Design review of the part built by this model. Coordinates are the model's own, in mm. Round coordinates to 2 decimals unless told otherwise and drop trailing zeros. Loops run counter-clockwise (first coordinate to the right, second up) from the corner with the lowest first, then second, coordinate; pieces in that order, holes last. Notation, with made-up numbers: (-33.5, -16.75) - (-1.5, -16.75) arc R19 cw to (-1.5, 13.25) - close; hole circle Ø7 at (76.25, -3). An arc over 180 degrees is marked (long way). Return JSON: item names as keys, results as strings. Group by question number.
(1) We need section C-C, the plane x = 113. Write out the cut boundary in (y, z).
(2) Wall thickness on L1, parallel to X at y = 10, z = 149.5; L2, parallel to Z at x = 57.5, y = -54.5; L3, parallel to Z at x = 42, y = 3.5: over which ranges is each line inside the solid? List them lowest first. Write a range as [from, to].
(3) We need section A-A, the plane x = 33.5. Write out the cut boundary in (y, z).
(4) Clearance check with flat-ended pins moving along their axes: pin 1 (10 mm diameter, centred on x = 6, y = -2.5, fed in from +Z); pin 2 (6 mm diameter, centred on y = 4, z = 160.5, fed in from -X); pin 3 (4.5 mm diameter, centred on x = 99, z = 153, fed in from -Y). State where each tip first meets the part, or that it passes through.
(5) We need section B-B, the plane y = -46. Write out the cut boundary in (x, z), and give its area (3 significant figures).
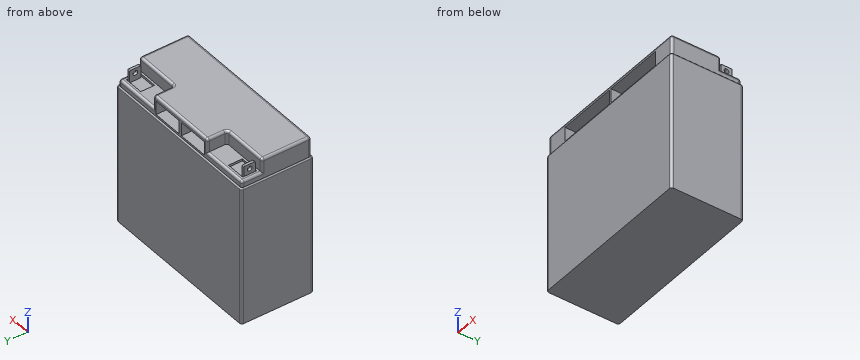
from build123d import *

# Parameters (mm, degrees)
SKETCH1_W                    = 177.8
SKETCH1_H                    = 146.05
BOSS_EXTRUDE1_DEPTH          = 76.2
SKETCH2_W                    = 174.845239449
SKETCH2_H                    = 73.245239449
BOSS_EXTRUDE2_DEPTH          = 21.082
SKETCH3_W                    = 14.224
SKETCH3_H                    = 21.336
CUT_EXTRUDE1_DEPTH           = 49.276
SKETCH4_W                    = 2.693561453
SKETCH4_H                    = 12
BOSS_EXTRUDE3_DEPTH          = 10.746
CUT_EXTRUDE2_DEPTH           = 2.254
SKETCH6_W                    = 49.276
SKETCH6_H                    = 14.224
CUT_EXTRUDE3_DEPTH           = 21.336
SKETCH7_W                    = 2.693561452
SKETCH7_H                    = 12
BOSS_EXTRUDE4_DEPTH          = 10.746
CUT_EXTRUDE4_DEPTH           = 2.254
SKETCH9_W                    = 33.02
SKETCH9_H                    = 14.399652357
CUT_EXTRUDE5_DEPTH           = 19.05
SKETCH10_W                   = 33.02
SKETCH10_H                   = 14.399652357
CUT_EXTRUDE6_DEPTH           = 19.05
SKETCH11_W                   = 63.5
SKETCH11_H                   = 15.201284342
CUT_EXTRUDE7_DEPTH           = 19.558
SKETCH12_W                   = 63.5
SKETCH12_H                   = 15.201284342
CUT_EXTRUDE8_DEPTH           = 19.558
F_5_0_5_DIAMETER_HOLE1_D     = 5
F_5_0_5_DIAMETER_HOLE1_DEPTH = 8.734014926
F_5_0_5_DIAMETER_HOLE2_D     = 5
F_5_0_5_DIAMETER_HOLE2_DEPTH = 8.734014926
FILLET1_R                    = 2.54
FILLET2_R                    = 1
FILLET3_R                    = 1.27


with BuildPart() as part:
    # Sketch1 → Boss-Extrude1 (new body)
    with BuildSketch(Plane.XZ.offset(62.213215728)):
        with Locations((55.786931477, 73.025)):
            Rectangle(SKETCH1_W, SKETCH1_H)
    extrude(amount=-BOSS_EXTRUDE1_DEPTH)

    # Sketch2 → Boss-Extrude2 (add)
    with BuildSketch(Plane.XY.offset(146.05)):
        with Locations((55.786931477, -24.113215728)):
            Rectangle(SKETCH2_W, SKETCH2_H)
    extrude(amount=BOSS_EXTRUDE2_DEPTH)

    # Sketch3 → Cut-Extrude1 (cut)
    with BuildSketch(Plane.ZY.offset(31.635688247)):
        with Locations((160.02, 1.841403997)):
            Rectangle(SKETCH3_W, SKETCH3_H)
    extrude(amount=-CUT_EXTRUDE1_DEPTH, mode=Mode.SUBTRACT)

    # Sketch4 → Boss-Extrude3 (add)
    with BuildSketch(Plane.XY.offset(152.908)):
        with Locations((-25.725834324, 0.632623113)):
            Rectangle(SKETCH4_W, SKETCH4_H)
    extrude(amount=BOSS_EXTRUDE3_DEPTH)

    # Sketch5 → Cut-Extrude2 (cut)
    with BuildSketch(Plane.XY.offset(152.908)):
        Polygon((-27.07261505, 6.632623113), (-24.379053597, 6.632623113), (-24.379053597, -5.367376887), (-27.07261505, -5.367376887), (-27.07261505, -6.677584717), (-6.787176985, -6.677584717), (-6.787176985, 7.942830943), (-27.07261505, 7.942830943), align=None)
    extrude(amount=-CUT_EXTRUDE2_DEPTH, mode=Mode.SUBTRACT)

    # Sketch6 → Cut-Extrude3 (cut)
    with BuildSketch(Plane(origin=(0, 12.509403997, 0), x_dir=(-1, 0, 0), z_dir=(0, 1, 0))):
        with Locations((-118.571551202, 160.02)):
            Rectangle(SKETCH6_W, SKETCH6_H)
    extrude(amount=-CUT_EXTRUDE3_DEPTH, mode=Mode.SUBTRACT)

    # Sketch7 → Boss-Extrude4 (add)
    with BuildSketch(Plane.XY.offset(152.908)):
        with Locations((137.299697278, 0.632623113)):
            Rectangle(SKETCH7_W, SKETCH7_H)
    extrude(amount=BOSS_EXTRUDE4_DEPTH)

    # Sketch8 → Cut-Extrude4 (cut)
    with BuildSketch(Plane.XY.offset(152.908)):
        Polygon((138.646478004, -5.367376887), (135.952916552, -5.367376887), (135.952916552, 6.632623113), (138.646478004, 6.632623113), (138.646478004, 7.942830943), (118.361039939, 7.942830943), (118.361039939, -6.677584717), (138.646478004, -6.677584717), align=None)
    extrude(amount=-CUT_EXTRUDE4_DEPTH, mode=Mode.SUBTRACT)

    # Sketch9 → Cut-Extrude5 (cut)
    with BuildSketch(Plane(origin=(0, 12.509403997, 0), x_dir=(-1, 0, 0), z_dir=(0, 1, 0))):
        with Locations((-73.820931477, 155.313650768)):
            Rectangle(SKETCH9_W, SKETCH9_H)
    extrude(amount=-CUT_EXTRUDE5_DEPTH, mode=Mode.SUBTRACT)

    # Sketch10 → Cut-Extrude6 (cut)
    with BuildSketch(Plane(origin=(0, 12.509403997, 0), x_dir=(-1, 0, 0), z_dir=(0, 1, 0))):
        with Locations((-37.752931477, 155.313650768)):
            Rectangle(SKETCH10_W, SKETCH10_H)
    extrude(amount=-CUT_EXTRUDE6_DEPTH, mode=Mode.SUBTRACT)

    # Sketch11 → Cut-Extrude7 (cut)
    with BuildSketch(Plane.XZ.offset(60.735835452)):
        with Locations((88.599551202, 155.2427389)):
            Rectangle(SKETCH11_W, SKETCH11_H)
    extrude(amount=-CUT_EXTRUDE7_DEPTH, mode=Mode.SUBTRACT)

    # Sketch12 → Cut-Extrude8 (cut)
    with BuildSketch(Plane.XZ.offset(60.735835452)):
        with Locations((22.974311753, 155.2427389)):
            Rectangle(SKETCH12_W, SKETCH12_H)
    extrude(amount=-CUT_EXTRUDE8_DEPTH, mode=Mode.SUBTRACT)

    # 5.0 _5_ Diameter Hole1
    with Locations(Plane.ZY.offset(-135.952916552)):
        with Locations((158.654, 0.632623113)):
            Hole(F_5_0_5_DIAMETER_HOLE1_D / 2, depth=F_5_0_5_DIAMETER_HOLE1_DEPTH)

    # 5.0 _5_ Diameter Hole2
    with Locations(Plane(origin=(-24.379053597, 0, 0), x_dir=(0, 0, -1), z_dir=(1, 0, 0))):
        with Locations((-158.654, 0.632623113)):
            Hole(F_5_0_5_DIAMETER_HOLE2_D / 2, depth=F_5_0_5_DIAMETER_HOLE2_DEPTH)

    # Fillet1
    fillet1_edges = [part.edges().sort_by_distance(p)[0] for p in [
        (144.686931477, 13.986784272, 73.025),
        (143.209551202, -60.735835452, 156.591),
        (-31.635688247, -60.735835452, 156.591),
        (143.209551202, -34.781215728, 167.132),
        (55.786931477, -60.735835452, 167.132),
        (-31.635688247, -34.781215728, 167.132),
        (-31.635688247, 12.509403997, 149.479),
        (17.640311753, 12.509403997, 160.02),
        (-6.997688247, 12.509403997, 152.908),
        (17.640311753, 1.841403997, 167.132),
        (17.640311753, -8.826596003, 160.02),
        (-6.997688247, -8.826596003, 167.132),
        (-31.635688247, 1.841403997, 152.908),
        (-31.635688247, -8.826596003, 160.02),
        (-33.113068523, 13.986784272, 73.025),
        (144.686931477, -62.213215728, 73.025),
        (-33.113068523, -62.213215728, 73.025),
        (55.786931477, 12.509403997, 167.132),
        (143.209551202, 12.509403997, 149.479),
        (143.209551202, -8.826596003, 160.02),
        (143.209551202, 1.841403997, 152.908),
        (118.571551202, -8.826596003, 167.132),
        (93.933551202, -8.826596003, 160.02),
        (93.933551202, 1.841403997, 167.132),
        (118.571551202, 12.509403997, 152.908),
        (93.933551202, 12.509403997, 160.02),
    ]]
    fillet(fillet1_edges, radius=FILLET1_R)

    # Fillet2
    fillet2_edges = [part.edges().sort_by_distance(p)[0] for p in [
        (-25.725834323, 6.632623113, 163.654),
        (-25.725834323, -5.367376887, 163.654),
        (137.299697278, 6.632623113, 163.654),
        (137.299697278, -5.367376887, 163.654),
    ]]
    fillet(fillet2_edges, radius=FILLET2_R)

    # Fillet3
    fillet3_edges = [part.edges().sort_by_distance(p)[0] for p in [
        (-33.113068523, -24.113215728, 146.05),
        (55.786931477, 13.986784272, 146.05),
        (55.786931477, -62.213215728, 146.05),
        (144.686931477, -24.113215728, 146.05),
        (143.942982701, 13.242835496, 146.05),
        (-32.369119747, -61.469266952, 146.05),
        (143.942982701, -61.469266952, 146.05),
        (-32.369119747, 13.242835496, 146.05),
    ]]
    fillet(fillet3_edges, radius=FILLET3_R)


solid = part.part
Solutions:
{
 "1": {"outline": "(-62.21, 0) - (13.99, 0) - (13.99, 144.78) arc R1.27 ccw to (12.72, 146.05) - (12.51, 146.05) - (12.51, 150.37) arc R2.54 ccw to (9.97, 152.91) - (-8.83, 152.91) - (-8.83, 164.59) arc R2.54 ccw to (-11.37, 167.13) - (-58.2, 167.13) arc R2.54 ccw to (-60.74, 164.59) - (-60.74, 162.84) - (-41.18, 162.84) - (-41.18, 147.64) - (-60.74, 147.64) - (-60.74, 146.05) - (-60.94, 146.05) arc R1.27 ccw to (-62.21, 144.78) - close"},
 "2": {"L1": "[-31.64, 21.24], [54.26, 57.31], [90.33, 143.21]", "L2": "[0, 147.64], [162.84, 167.13]", "L3": "[0, 148.11], [162.51, 167.13]"},
 "3": {"outline": "(-62.21, 0) - (13.99, 0) - (13.99, 144.78) arc R1.27 ccw to (12.72, 146.05) - (12.51, 146.05) - (12.51, 148.11) - (-6.54, 148.11) - (-6.54, 162.51) - (12.51, 162.51) - (12.51, 164.59) arc R2.54 ccw to (9.97, 167.13) - (-58.2, 167.13) arc R2.54 ccw to (-60.74, 164.59) - (-60.74, 162.84) - (-41.18, 162.84) - (-41.18, 147.64) - (-60.74, 147.64) - (-60.74, 146.05) - (-60.94, 146.05) arc R1.27 ccw to (-62.21, 144.78) - close"},
 "4": {"pin 1": "z = 152.91", "pin 2": "x = -27.07", "pin 3": "y = -41.18"},
 "5": {"outline": "(-33.11, 0) - (144.69, 0) - (144.69, 144.78) arc R1.27 ccw to (143.42, 146.05) - (143.21, 146.05) - (143.21, 164.59) arc R2.54 ccw to (140.67, 167.13) - (-29.1, 167.13) arc R2.54 ccw to (-31.64, 164.59) - (-31.64, 146.05) - (-31.84, 146.05) arc R1.27 ccw to (-33.11, 144.78) - close; hole (-8.78, 147.64) - (54.72, 147.64) - (54.72, 162.84) - (-8.78, 162.84) - close; hole (56.85, 147.64) - (120.35, 147.64) - (120.35, 162.84) - (56.85, 162.84) - close", "area": "27,700 mm^2"}
}
